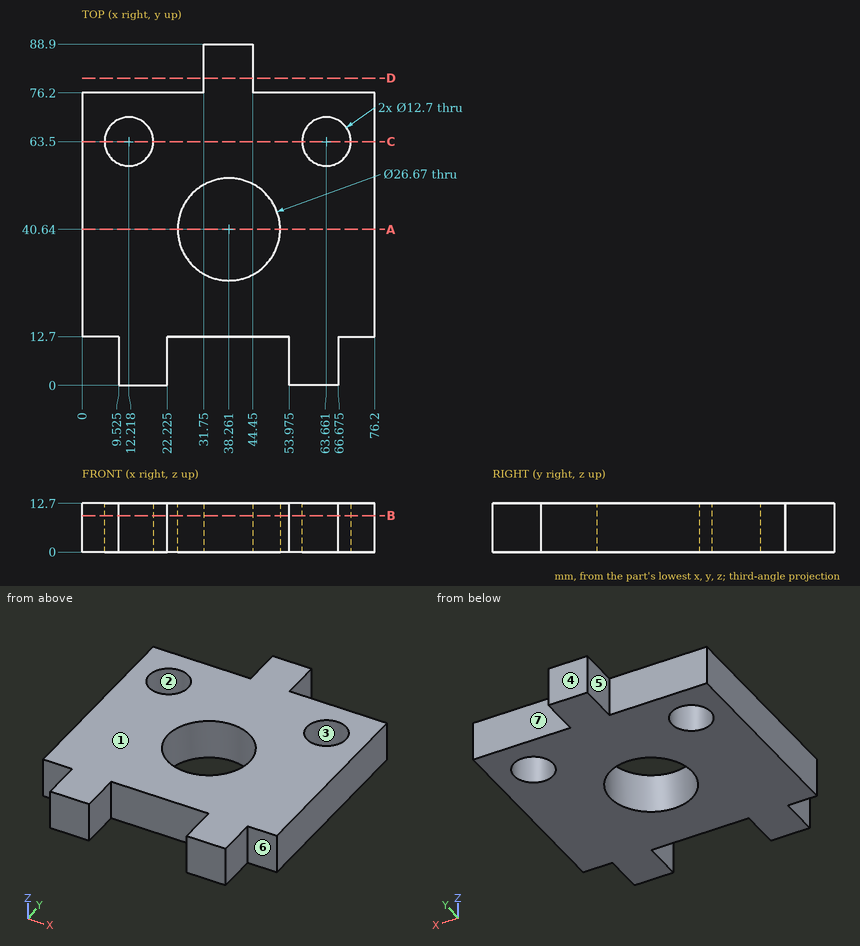
Design review of the part shown in the three views and the two pictorial views. Dimensions are in mm from the part's minimum x, y and z. A direction names the side the tool comes from. Coordinates: 2 decimals unless noted, no trailing zeros. Loops run counter-clockwise (first coordinate to the right, second up) from the corner with the lowest first, then second, coordinate; pieces in that order, holes last. Notation, with made-up numbers: M 47.5,-1 L 64.5,-1 A32 ccw 64.5,25 Z; hole C 11.25,34.5 d6. An arc over 180 degrees is marked long. One line per question, with ' | ' between items.
(1) We need section D-D (y = 80). Give the boundary of the cut face in (x, z).
Filled in:
outline: M 31.75,0 L 44.45,0 L 44.45,12.7 L 31.75,12.7 Z
(2) We need section B-B (z = 9.5). Count the separate pieces of the cut face and the enclosed holes in it, and give its area (3 significant figures).
Filled in:
separate pieces: 1 | enclosed holes: 3 | area: 4,510 mm^2
(3) Draft analysis for pull direction Y (two halves, no side actions). For the marked faces 1, 2, 3 and 4, state which applies: released by +Y, released by -Y, zero draft, split by the parting line, or undercut.
Filled in:
face 1: zero draft | face 2: undercut | face 3: undercut | face 4: released by +Y
(4) Wall thickness on probe 1 along X at (y, z) = (7, 2.5) (1 decimal); probe 2 along X at (y, z) = (65, 11.5); probe 3 along Y at (x, z) = (64, 10.5): over which ranges is each line inside the solid? List them lowest first.
Filled in:
probe 1: x = 9.5 to 22.2, 54 to 66.7 | probe 2: x = 0 to 6.05, 18.39 to 57.49, 69.83 to 76.2 | probe 3: y = 0 to 57.16, 69.84 to 76.2
(5) For pin 1 Ø1 at (x, y) = (42, 51.5) entering from -Z; pin 2 Ø6 at (x, z) = (59, 3) entering from -Y; pin 3 Ø6.5 at (x, z) = (46, 3) entering from -Y; pin 4 Ø4 at (x, z) = (8, 6) entering from +Y, all flat-tipped, find the tip position at first contact; note any pin that passes through.
Filled in:
pin 1: passes through | pin 2: stops at y = 0 | pin 3: stops at y = 12.7 | pin 4: stops at y = 76.2
(6) We need section A-A (y = 40.64). Give the boundary of the cut face in (x, z) (1 decimal).
Filled in:
outline: M 0,0 L 24.9,0 L 24.9,12.7 L 0,12.7 Z; M 51.6,0 L 76.2,0 L 76.2,12.7 L 51.6,12.7 Z
(7) Machinability: for the marked faces 5, 6 and 7, which of the approach directions +Z, -Z, +X, -X, +Y, -Y give a long, thin tool a straight path to every point of the face, cutting with its end or side? Answer none if there is none.
Filled in:
face 5: +Z, -Z, -X, +Y | face 6: +Z, -Z, +X, -Y | face 7: +Z, -Z, +X, +Y
(8) We need section C-C (y = 63.5). Give the boundary of the cut face in (x, z).
Filled in:
outline: M 0,0 L 5.87,0 L 5.87,12.7 L 0,12.7 Z; M 18.57,0 L 57.31,0 L 57.31,12.7 L 18.57,12.7 Z; M 70.01,0 L 76.2,0 L 76.2,12.7 L 70.01,12.7 Z
